Autodesk Inventor part; units mm, degrees
ref_plane "우측면도" through (0, 0, 0) normal (1, 0, 0) x (0, 1, 0)
ref_plane "평면도" through (0, 0, 0) normal (0, 1, 0) x (-1, 0, 0)
ref_plane "정면도" through (0, 0, 0) normal (0, 0, 1) x (1, 0, 0)
sketch "스케치1" plane through (0, 0, 0) normal (0, 1, 0) x (-1, 0, 0)
  line L0 (0, 0) -> (0, -100)
  line L1 (0, -100) -> (-50, -100)
  line L2 (-50, -100) -> (-50, 0)
  line L3 (-50, 0) -> (0, 0)
  line L4 (2.5, -102.5) -> (2.5, 2.5)
  line L5 (2.5, 2.5) -> (-52.5, 2.5)
  line L6 (-52.5, 2.5) -> (-52.5, -102.5)
  line L7 (-52.5, -102.5) -> (2.5, -102.5)
  line L8 (1, -101) -> (1, 1)
  line L9 (1, 1) -> (-51, 1)
  line L10 (-51, 1) -> (-51, -101)
  line L11 (-51, -101) -> (1, -101)
  line L12 (1.5, -101.5) -> (1.5, 1.5)
  line L13 (1.5, 1.5) -> (-51.5, 1.5)
  line L14 (-51.5, 1.5) -> (-51.5, -101.5)
  line L15 (-51.5, -101.5) -> (1.5, -101.5)
  dimension "d1" = 50
  dimension "d2" = 100
  dimension "d5" = 2.5
  dimension "d6" = 1.5
  dimension "d7" = 0.5
extrude "돌출1" add sketch "스케치1" along normal blind 34 contours L7 L6 L5 L4 | L11 L10 L9 L8 | L15 L14 L13 L12
sketch "스케치4" plane through (50, 0, 0) normal (-1, 0, 0) x (0, 0, 1)
  line L0 (-100, 34) -> (0, 34)
  line L1 (-100, 34) -> (0, 34)
  line L2 (0, 34) -> (0, 31.5)
  line L3 (0, 31.5) -> (-100, 31.5)
  line L4 (-100, 34) -> (-100, 31.5)
  line L5 (0, 34) -> (0, 31.5)
  point P0 (0, 0)
  dimension "d12" = 2.5
sketch "스케치5" plane through (0, 0, -100) normal (1, 0, 0) x (0, 0, -1)
  line L0 (-100, 34) -> (0, 34)
  line L1 (0, 34) -> (0, 31.5)
  line L2 (0, 31.5) -> (-100, 31.5)
  line L3 (-100, 34) -> (-100, 31.5)
  line L4 (-100, 34) -> (0, 34)
  point P0 (-100, 0)
  dimension "d13" = 2.5
loft "로프트1" add profiles "스케치4", "스케치5"
sketch "스케치6" plane through (0, 34, 0) normal (0, 1, 0) x (1, 0, 0)
  line L0 (-2.5, 102.5) -> (-2.5, -2.5)
  line L1 (-2.5, -2.5) -> (52.5, -2.5)
  line L2 (52.5, -2.5) -> (52.5, 102.5)
  line L3 (52.5, 102.5) -> (-2.5, 102.5)
  circle A0 centre (25, 50) radius 6
  point P0 (0, 0)
  dimension "d18" = 12
  dimension "d31" = 27.5
  dimension "d32" = 52.5
extrude "돌출2" cut sketch "스케치6" against normal blind 50 contours A0
sketch "스케치8" plane through (0, 0, 0) normal (0, -1, 0) x (1, 0, 0)
  line L0 (50, -100) -> (0, -100)
  line L1 (0, -100) -> (0, 0)
  line L2 (0, 0) -> (50, 0)
  line L3 (50, 0) -> (50, -100)
  line L4 (-2.5, -102.5) -> (-2.5, 2.5)
  line L5 (52.5, -102.5) -> (-2.5, -102.5)
  line L6 (52.5, 2.5) -> (52.5, -102.5)
  line L7 (-2.5, 2.5) -> (52.5, 2.5)
  line L8 (-1.5, -101.5) -> (-1.5, 1.5)
  line L9 (-1, -101) -> (-1, 1)
  line L10 (-1.5, 1.5) -> (51.5, 1.5)
  line L11 (-1, 1) -> (51, 1)
  line L12 (51, 1) -> (51, -101)
  line L13 (51.5, 1.5) -> (51.5, -101.5)
  line L14 (51, -101) -> (-1, -101)
  line L15 (51.5, -101.5) -> (-1.5, -101.5)
extrude "돌출4" cut sketch "스케치8" against normal blind 2.5 contours L8 L10 L13 L15
sketch "스케치9" plane through (52.5, 0, 2.5) normal (1, 0, 0) x (0, 0, -1)
  line L0 (0, 0) -> (105, 0)
  line L1 (105, 0) -> (105, 34)
  line L2 (0, 34) -> (105, 34)
  line L3 (0, 0) -> (0, 34)
  line L4 (7.5, 11.5) -> (18.5, 11.5)
  line L5 (18.5, 11.5) -> (18.5, 5)
  line L6 (18.5, 5) -> (7.5, 5)
  line L7 (7.5, 5) -> (7.5, 11.5)
  point P0 (2.5, 0)
  dimension "d25" = 6.5
  dimension "d26" = 11
  dimension "d27" = 5
  dimension "d28" = 5
extrude "돌출5" cut sketch "스케치9" against normal blind 10 contours L4 L5 L6 L7
properties part number "호출벨 new"
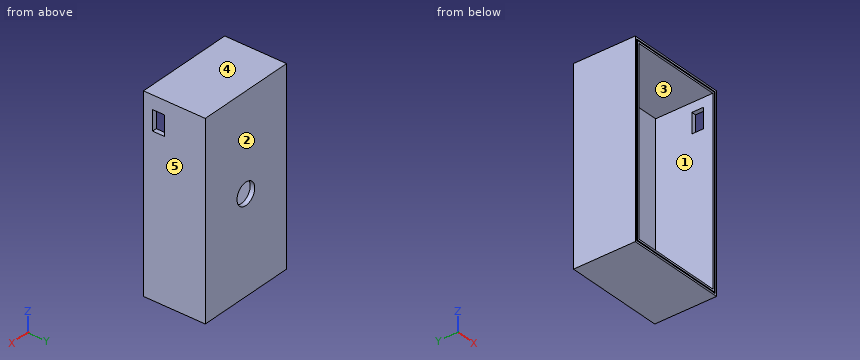
Verification items for the finished model (mm, model axes). Face numbers are marked on the shaded views. A direction names the side the tool comes from. Give positions to 0.01 mm unless a question says otherwise; leave off trailing zeros. Order: outer loops, then holes, each group sorted by start corner. A loop starts at its lowest first (then second) coordinate and runs counter-clockwise, first axis right, second up. Notation, with made-up numbers: M 46.5,-14.5 L 64.5,-14.5 A9 cw 64.5,-4.5 Z; hole C 73.5,3.5 d5. An arc over 180 degrees is marked long. Use one line per item in the form item = value. Start each with the question number.
Q1. Access from +Z, -Z, +X, -X, +Y, -Y to the whole of each face (thin tool, end or side, straight path). Record for the marked faces 1 and 2.
Q2. Section check B-B (x = 25). Enter the section's corners in (y, z), then the cut area to 4 significant figures.
Q3. Section check C-C (y = 3.5). Enter the section's corners in (x, z), then the cut area to 3 significant figures.
Q4. Section check A-A (z = -50). Enter the section's corners in (x, y).
Q5. Mould release check, pull along X, two halves, no side actions. Record for the marked faces 3, 4 and 5: +X half, -X half, draft (parallel to the pull), parting line (faces both ways), or undercut.
Q6. Section check D-D (x = 17.5). Enter the section's corners in (y, z).
Q7. Go/stop test with flat-tipped pins: pin 1 Ø1 at (x, z) = (31, -51) entering from -Y; pin 2 Ø3 at (x, z) = (51, -12) entering from -Y. Record where each tip stops, or that it passes through.
Q8. Scan lines: line 1 along Z through (x, y) = (18.5, 18); line 2 along X through (y, z) = (33, -50); line 3 along X through (y, z) = (5.5, -51.5). Record each from-to range of solid material in increasing order. Write a range as [from, to].
Evaluation:
q1.face_1 = -Y
q1.face_2 = +Z, -Z, +X, -X, +Y
q2.outline = M 0,-102.5 L 34,-102.5 L 34,-56 L 31.5,-56 L 31.5,-100 L 0,-100 L 0,-101 L 2.5,-101 L 2.5,-101.5 L 0,-101.5 Z; M 0,0 L 31.5,0 L 31.5,-44 L 34,-44 L 34,2.5 L 0,2.5 L 0,1.5 L 2.5,1.5 L 2.5,1 L 0,1 Z
q2.area = 387.5 mm2
q3.outline = M -2.5,-102.5 L 52.5,-102.5 L 52.5,2.5 L -2.5,2.5 Z; hole M 0,-100 L 50,-100 L 50,0 L 0,0 Z
q3.area = 775 mm2
q4.outline = M -2.5,0 L -1.5,0 L -1.5,2.5 L -1,2.5 L -1,0 L 0,0 L 0,31.5 L 19,31.5 L 19,34 L -2.5,34 Z; M 31,31.5 L 50,31.5 L 50,0 L 51,0 L 51,2.5 L 51.5,2.5 L 51.5,0 L 52.5,0 L 52.5,34 L 31,34 Z
q5.face_3 = undercut
q5.face_4 = draft
q5.face_5 = +X half
q6.outline = M 0,-102.5 L 34,-102.5 L 34,2.5 L 0,2.5 L 0,1.5 L 2.5,1.5 L 2.5,1 L 0,1 L 0,0 L 31.5,0 L 31.5,-100 L 0,-100 L 0,-101 L 2.5,-101 L 2.5,-101.5 L 0,-101.5 Z
q7.pin_1 = 31.5
q7.pin_2 = 0
q8.line_1 = [-102.5, -100], [0, 2.5]
q8.line_2 = [-2.5, 19], [31, 52.5]
q8.line_3 = [-2.5, 0], [50, 52.5]
